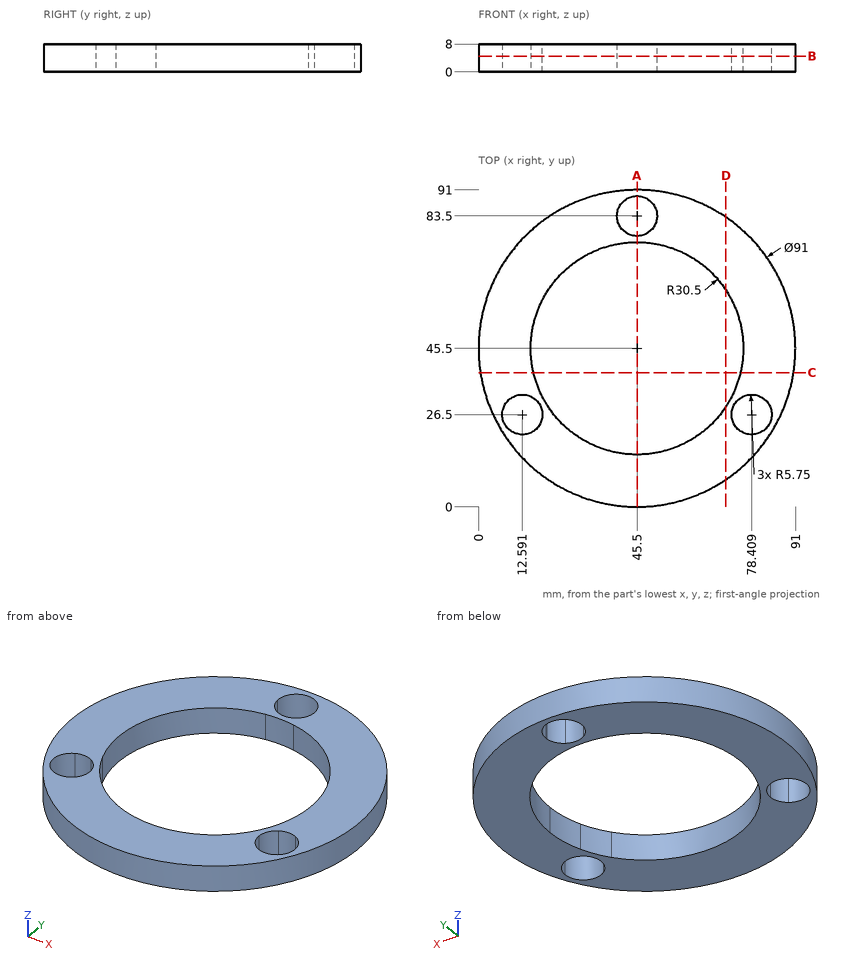
Study the drawing (mm; zero at the part's minimum x, y, z) and answer. Coordinates: 2 decimals unless noted, no trailing zeros. Write each loop counter-clockwise with the first axis right and the second up, starting at its lowest first coordinate (ties: lowest second). Pieces come first, ordered by that corner, then holes. Notation, with made-up numbers: (-4, 22.25) - (54, 22.25) arc R20 cw to (54, 57.25) - close; hole circle Ø4 at (83, 53.5). An arc over 180 degrees is marked (long way). Return JSON: item names as keys, results as strings. Group by question number.
1. Straight lines are drawn through the part: L1, parallel to Y at x = 40.5, z = 6.5; L2, parallel to X at y = 63, z = 6.5; L3, parallel to Y at x = 82, z = 1.75. For each, find the intervals that lie inside material, in ascending order.
2. A cutting plane is placed at A-A, the plane x = 45.5. Determine the outline of the cut face in (y, z).
3. Given pin 1 (3 mm diameter, centred on x = 32.5, z = 3, fed in from +Y); pin 2 (4 mm diameter, centred on y = 75, z = 6.5, fed in from +X); pin 3 (6 mm diameter, centred on x = 35.5, y = 22.5, fed in from +Z), each flat-ended and moving along its own axis, determine where each tip first touches the part or whether it passes through.
4. A cutting plane is placed at D-D, the plane x = 71. Determine the outline of the cut face in (y, z), plus the area to 3 significant figures.
5. A cutting plane is placed at B-B, the plane z = 4.5. Give the number of separate pieces and of enclosed holes in the cut face, plus the area to 3 significant figures.
6. A cutting plane is placed at C-C, the plane y = 38.5. Determine the outline of the cut face in (x, z), plus the area to 3 significant figures.
Ans:
{
 "1": {"L1": "0.28 to 15.41, 75.59 to 80.66, 86.34 to 90.72", "L2": "3.5 to 20.52, 70.48 to 87.5", "L3": "18.33 to 22.01, 30.99 to 72.67"},
 "2": {"outline": "(0, 0) - (15, 0) - (15, 8) - (0, 8) - close; (76, 0) - (77.75, 0) - (77.75, 8) - (76, 8) - close; (89.25, 0) - (91, 0) - (91, 8) - (89.25, 8) - close"},
 "3": {"pin 1": "y = 89.52", "pin 2": "x = 81.75", "pin 3": "through"},
 "4": {"outline": "(7.82, 0) - (28.77, 0) - (28.77, 8) - (7.82, 8) - close; (62.23, 0) - (83.18, 0) - (83.18, 8) - (62.23, 8) - close", "area": "335 mm²"},
 "5": {"separate pieces": "1", "enclosed holes": "4", "area": "3,270 mm²"},
 "6": {"outline": "(0.54, 0) - (15.81, 0) - (15.81, 8) - (0.54, 8) - close; (75.19, 0) - (90.46, 0) - (90.46, 8) - (75.19, 8) - close", "area": "244 mm²"}
}
